Can you work these out from the model? Positions are in its coordinate system, mm. A direction names the side the tool comes from. Coordinates: 2 decimals unless noted, no trailing zeros. Order: outer loops, then holes, each group sorted by start corner. A loop starts at its lowest first (then second) coordinate and runs counter-clockwise, first axis right, second up. Notation, with made-up numbers: (10.5, 40.5) -> (16.5, 40.5) arc R25 ccw to (16.5, 75.5) -> close; hole circle Ø1 at (26, 0.25). An arc over 180 degrees is marked (long way). Return JSON: item names as keys, results as strings. Group by question number.
1) If we section it at B-B, the plane z = -6: Please give me the cut outline in (x, y).
2) For pin 1 (4 mm diameter, centred on y = -415, z = 1.5, fed in from -X); pin 2 (5 mm diameter, centred on x = 1.6, y = 647.7, fed in from -Z); pin 3 (10 mm diameter, centred on x = 1.6, y = -622.3, fed in from +Z) (3 decimals); pin 4 (1.9 mm diameter, centred on y = -588.5, z = 22.5, fed in from -X), each with a flat end and sliding along its axis, tell me the tip position at first contact or that it passes through.
3) If we section it at A-A, the plane y = 464: Please give me the cut outline in (x, z), then the cut area to 3 significant figures.
4) For faces 1 (the flat face through (-4, -9, 19.05)), 2 (the flat face through (-4, -609, 22.225)), 3 (the flat face through (-4, 610, 22.225)), 4 (the flat face through (18, 660.4, 6)), 5 (the flat face through (0, -9, 25.4)), which set-ups out of +Z, -Z, +X, -X, +Y, -Y let a thin tool reach every point of the face, with its end or its side?
5) If I drill on probe 1 along Y at (x, z) = (2, 19.5); probe 2 along X at (y, z) = (647.7, 20.9); probe 3 along X at (y, z) = (622.3, 19.8), over which ranges is the centre line in solid material (lowest first)? Write a range as from..to.
from build123d import *

# Parameters (mm, degrees)
F1_DEPTH = 660.4
F2_W     = 30.1752
F2_H     = 101.6
F2_R     = 3.175
F3_DEPTH = 3.175
F4_D     = 6.35
F5_DEPTH = 49.2135


with BuildPart() as f1:
    # F0 (on Front) → F1 (new body, symmetric)
    with BuildSketch(Plane.XZ):
        Polygon((17.4625, -23.812496), (23.8125, -23.812496), (23.8125, 25.400004), (-25.4, 25.400004), (-25.4, 19.050004), (17.4625, 19.050004), align=None)
    extrude(amount=F1_DEPTH, both=True)

    # F2 (on face) → F3 (cut)
    with BuildSketch(Plane.XY.offset(25.400004)):
        with Locations((-3.9624, -609.6)):
            Rectangle(F2_W, F2_H)
        with Locations((-9.525, -647.7)):
            Circle(F2_R, mode=Mode.SUBTRACT)
        with Locations((-9.525, -596.9)):
            Circle(F2_R, mode=Mode.SUBTRACT)
        with Locations((1.6002, -622.3)):
            Circle(F2_R, mode=Mode.SUBTRACT)
        with Locations((1.6002, -571.5)):
            Circle(F2_R, mode=Mode.SUBTRACT)
        with Locations((-3.9624, 609.6)):
            Rectangle(F2_W, F2_H)
        with Locations((-9.525, 571.5)):
            Circle(F2_R, mode=Mode.SUBTRACT)
        with Locations((-9.525, 622.3)):
            Circle(F2_R, mode=Mode.SUBTRACT)
        with Locations((1.6002, 596.9)):
            Circle(F2_R, mode=Mode.SUBTRACT)
        with Locations((1.6002, 647.7)):
            Circle(F2_R, mode=Mode.SUBTRACT)
    extrude(amount=-F3_DEPTH, mode=Mode.SUBTRACT)

    # F4 (through all)
    with Locations(Plane.XY.offset(25.400004)):
        with Locations((1.6002, -571.5), (-9.525, -596.9), (1.6002, -622.3), (-9.525, -647.7), (1.6002, 647.7), (-9.525, 622.3), (1.6002, 596.9), (-9.525, 571.5)):
            Hole(F4_D / 2)

    # F2 (on face) → F5 (cut, through all)
    with BuildSketch(Plane.XY.offset(25.400004)):
        Polygon((-25.4, 660.4), (-25.4, 552.5516), (-19.05, 552.5516), (-19.05, 558.8), (-19.05, 660.4), align=None)
        Polygon((-19.05, -552.5516), (-25.4, -552.5516), (-25.4, -660.4), (-19.05, -660.4), (-19.05, -558.8), align=None)
    extrude(amount=-F5_DEPTH, mode=Mode.SUBTRACT)


solid = f1.part
Result sheet:
{
 "1": {"outline": "(17.46, -660.4) -> (23.81, -660.4) -> (23.81, 660.4) -> (17.46, 660.4) -> close"},
 "2": {"pin 1": "stops at x = 17.46", "pin 2": "passes through", "pin 3": "stops at z = 22.225", "pin 4": "stops at x = -19.05"},
 "3": {"outline": "(-25.4, 19.05) -> (17.46, 19.05) -> (17.46, -23.81) -> (23.81, -23.81) -> (23.81, 25.4) -> (-25.4, 25.4) -> close", "area": "585 mm2"},
 "4": {"face 1": "-Z, -X, +Y, -Y", "face 2": "+Z, -X, -Y", "face 3": "+Z, -X, +Y", "face 4": "+Z, -Z, +X, -X, +Y", "face 5": "+Z, +X, -X, +Y, -Y"},
 "5": {"probe 1": "y = -660.4..-625.45, -619.15..-574.65, -568.35..593.75, 600.05..644.55, 650.85..660.4", "probe 2": "x = -19.05..-1.57, 4.78..23.81", "probe 3": "x = -19.05..-12.7, -6.35..23.81"}
}
